Autodesk Inventor part; units mm, degrees
ref_plane "YZ Plane" through (0, 0, 0) normal (1, 0, 0) x (0, 1, 0)
ref_plane "XZ Plane" through (0, 0, 0) normal (0, 1, 0) x (-1, 0, 0)
ref_plane "XY Plane" through (0, 0, 0) normal (0, 0, 1) x (1, 0, 0)
sketch "Skizze1" plane through (0, 0, 0) normal (0, 1, 0) x (-1, 0, 0)
  line L0 (-15, 30) -> (15, 30)
  line L1 (15, 30) -> (15, -30)
  line L2 (15, -30) -> (-15, -30)
  line L3 (-15, -30) -> (-15, 30)
  line L4 (-15, 30) -> (15, -30) construction
  line L5 (15, 30) -> (-15, -30) construction
  point P0 (0, 0)
  dimension "d0" = 30
  dimension "d1" = 60
extrude "Extrusion1" add sketch "Skizze1" along normal mid plane 30
sketch "Skizze3" plane through (0, 15, 0) normal (0, 1, 0) x (1, 0, 0)
  line L0 (15, -15) -> (-15, -15)
  line L1 (-15, -15) -> (-15, 15)
  line L2 (-15, 15) -> (15, 15)
  line L3 (15, 15) -> (15, -15)
  line L4 (15, -15) -> (-15, 15) construction
  line L5 (-15, -15) -> (15, 15) construction
  point P0 (0, 0)
  dimension "d11" = 30
  dimension "d12" = 30
extrude "Extrusion2" cut sketch "Skizze3" against normal blind 15
sketch "Skizze4" plane through (-15, 15, 30) normal (0, 0, 1) x (1, 0, 0)
  circle A0 centre (15, -15) radius 0.8
  dimension "d15" = 1.6
hole "Kapillare" at (0, 0, 30) direction (0, 0, -1) diameter 1.6 end through all
sketch "Skizze5" plane through (0, -15, 0) normal (0, -1, 0) x (1, 0, 0)
  circle A0 centre (0, 0) radius 0.4
  dimension "d23" = 0.8
hole "Bohrung3" at (0, -15, 0) direction (0, 1, 0) diameter 0.8 end through all
sketch "Skizze6" plane through (15, 15, -30) normal (0, 0, -1) x (-1, 0, 0)
  point P0 (15, -15)
  point P1 (15, -15)
hole "Bohrung4" at (0, 0, -30) direction (0, 0, 1) diameter 5.5 depth 5.7
sketch "Skizze7" plane through (-15, 15, 30) normal (0, 0, 1) x (1, 0, 0)
  point P0 (15, -15)
  point P1 (15, -15)
hole "Bohrung5" at (0, 0, 30) direction (0, 0, -1) diameter 5.5 depth 5.7
sketch "Skizze8" plane through (0, -15, 0) normal (0, -1, 0) x (1, 0, 0)
  point P0 (0, 0)
  point P1 (0, 0)
hole "Bohrung6" at (0, -15, 0) direction (0, 1, 0) diameter 5.5 depth 5.7
sketch "Skizze17" plane through (0, -15, 0) normal (0, -1, 0) x (1, 0, 0)
  line L0 (10.5, 10.5) -> (-10.5, 10.5)
  line L1 (-10.5, 10.5) -> (-10.5, -10.5)
  line L2 (-10.5, -10.5) -> (10.5, -10.5)
  line L3 (10.5, -10.5) -> (10.5, 10.5)
  circle A0 centre (0, 0) radius 0.4
  line L4 (10.5, 10.5) -> (-10.5, -10.5) construction
  line L5 (-10.5, 10.5) -> (10.5, -10.5) construction
  dimension "d60" = 21
  dimension "d61" = 21
hole "Bohrung8" at (10.5, -15, -10.5) at (-10.5, -15, -10.5) at (10.5, -15, 10.5) at (-10.5, -15, 10.5) direction (0, 1, 0) diameter 3 end through all
sketch "Skizze18" plane through (0, -15, 0) normal (0, -1, 0) x (1, 0, 0)
  point P0 (0, 0)
properties part number "LS1_Basis" material "PMMA-Kunststoff"
Build history of the part. All positions in model axes, mm. A direction names the side the tool comes from. Round coordinates to 2 decimals unless told otherwise and drop trailing zeros. Write each loop counter-clockwise with the first axis right and the second up, starting at its lowest first coordinate (ties: lowest second). Pieces come first, ordered by that corner, then holes. Notation, with made-up numbers: M 81.5,28 L 114.5,28 A20 ccw 114.5,61 Z; hole C -37.75,29.5 d9. An arc over 180 degrees is marked long. Answer as a JSON object with one key per item and string values. Group by question number.
(1) Which spindle directions (+Z, -Z, +X, -X, +Y, -Y) get a long thin tool onto all of the face, cutting with end or side? Do faces 1 (the flat face through (0, 8, 15)), 2 (the flat face through (0, 15, 23)), 3 (the flat face through (1, 1, -24.3)), 4 (the cylindrical face through (2.685, -12.11, 0.596)), 5 (the flat face through (1, -1, 24.3)). Say none if no direction does.
(2) Cut at B-B (y = 8.5). Give the cut face in (x, z).
(3) Mould opens along Y. For faces 6 (the flat face through (4, -15, 0)), 7 (the cylindrical face through (11.4, -7.4, -9.3)), 8 (the cylindrical face through (2.685, -0.596, -27.11)) say: pulls with the +Y half, pulls with the -Y half, needs draft (parallel to the pull), parting line crosses it, or undercut.
(4) Flat gauge pins, fed straight in: pin 1 (4.5 mm diameter, centred on x = 0, y = 0, fed in from -Z); pin 2 (3.5 mm diameter, centred on x = 0, y = 0, fed in from +Z); pin 3 (7 mm diameter, centred on x = 6.5, z = -0.5, fed in from +Y). Where does each tip first touch, or does it go through?
(5) Drill centre lines: L1, parallel to Z at x = -10.5, y = -12; L2, parallel to X at y = -6.75, z = -10.5; L3, parallel to Z at x = 9.5, y = 13.5. Where is each one in solid material? Low to high.
(6) Cut at A-A (x = -10.5). Give the cut face in (y, z), and give its area (3 significant figures).
(7) Cut at D-D (y = -10.5). Give the cut face in (x, z).
(8) Cut at C-C (z = 11). Give the cut face in (x, y).
Responses:
{
 "1": {"face 1": "+X, -X, +Y", "face 2": "+Z, -Z, +X, -X, +Y", "face 3": "-Z", "face 4": "-Y", "face 5": "+Z"},
 "2": {"outline": "M -15,-30 L 15,-30 L 15,-15 L -15,-15 Z; M -15,15 L 15,15 L 15,30 L -15,30 Z"},
 "3": {"face 6": "pulls with the -Y half", "face 7": "needs draft", "face 8": "undercut"},
 "4": {"pin 1": "stops at z = -24.3", "pin 2": "stops at z = 24.3", "pin 3": "stops at y = 0"},
 "5": {"L1": "z = -30 to -12, -9 to 9, 12 to 30", "L2": "x = -15 to -12, -9 to 9, 12 to 15", "L3": "z = -30 to -15, 15 to 30"},
 "6": {"outline": "M -15,-30 L 15,-30 L 15,-15 L 0,-15 L 0,-12 L -15,-12 Z; M -15,-9 L 0,-9 L 0,9 L -15,9 Z; M -15,12 L 0,12 L 0,15 L 15,15 L 15,30 L -15,30 Z", "area": "1,260 mm2"},
 "7": {"outline": "M -15,-30 L 15,-30 L 15,30 L -15,30 Z; hole C -10.5,-10.5 d3; hole C -10.5,10.5 d3; hole C 0,0 d5.5; hole C 10.5,-10.5 d3; hole C 10.5,10.5 d3"},
 "8": {"outline": "M -15,-15 L -11.91,-15 L -11.91,0 L -15,0 Z; M -9.09,-15 L 9.09,-15 L 9.09,0 L 0.8,0 A0.8 cw -0.8,0 L -9.09,0 Z; M 11.91,-15 L 15,-15 L 15,0 L 11.91,0 Z"}
}
